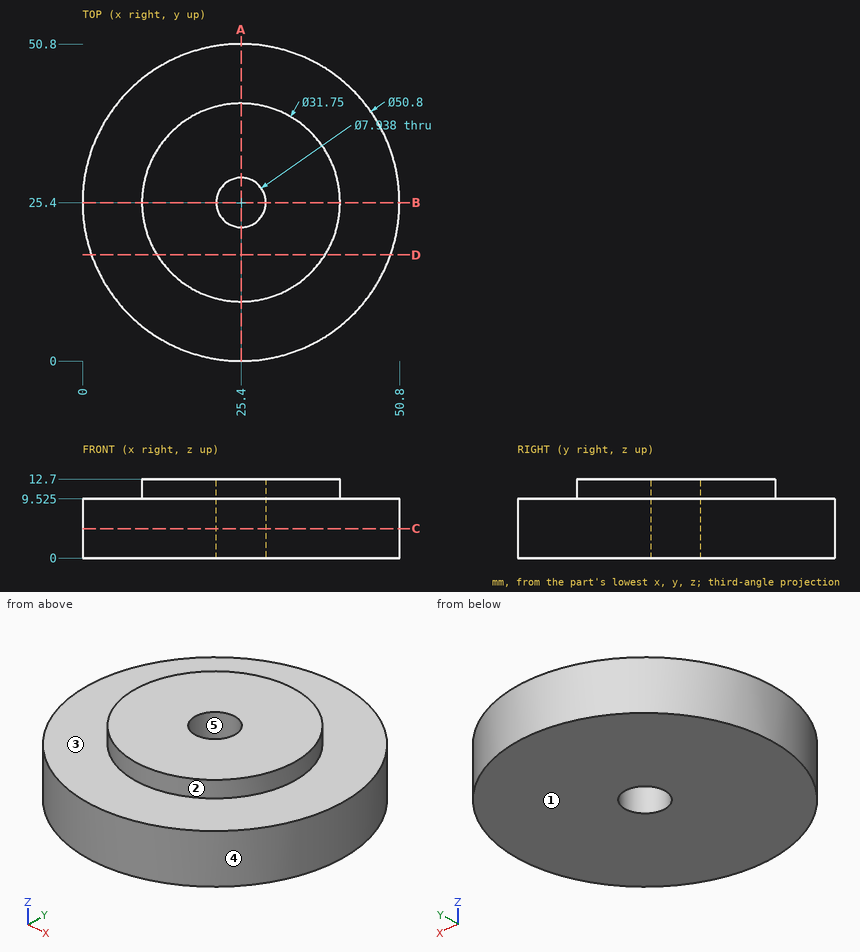
Print and shaded views of the part. All mm, measured from the part's lowest x, y and z. A direction names the side the tool comes from. Coordinates: 2 decimals unless noted, no trailing zeros. Order: outer loops, then holes, each group sorted by start corner. A loop starts at its lowest first (then second) coordinate and runs counter-clockwise, first axis right, second up. Notation, with made-up numbers: (-11.5, 38) - (33.5, 38) arc R27 cw to (33.5, 54) - close; hole circle Ø9 at (62, 49). An arc over 180 degrees is marked (long way). Return JSON: item names as keys, results as strings. Group by question number.
Item 1: Pin check, flat tips, straight feed: pin 1 (3 mm diameter, centred on x = 8.5, z = 7.5, fed in from -Y); pin 2 (1 mm diameter, centred on x = 26, z = 10.5, fed in from -Y) (1 decimal); pin 3 (5 mm diameter, centred on y = 39.5, z = 3.5, fed in from +X). Stop position of each tip, or through.
Item 2: Cut at C-C (z = 4.75). List the corners of the cut face in (x, y).
Item 3: Cut at D-D (y = 17). List the corners of the cut face in (x, z) (1 decimal).
Item 4: Which spindle directions (+Z, -Z, +X, -X, +Y, -Y) get a long thin tool onto all of the face, cutting with end or side? Do the marked faces 1 and 2. Say none if no direction does.
Item 5: Pull direction Y, two halves, no side cores. Call the marked faces 3, 4 and 5: pulls with the +Y half, pulls with the -Y half, needs draft (parallel to the pull), parting line crosses it, or undercut.
Item 6: Drill centre lines: probe 1 along Y at (x, z) = (25.4, 3.25); probe 2 along Z at (x, y) = (47, 31.5) (1 decimal); probe 3 along Y at (x, z) = (25.4, 10) (1 decimal). Where is each one in solid material? Low to high. Write a range as from..to.
Item 7: Cut at A-A (x = 25.4). List the corners of the cut face in (y, z) (1 decimal).
Check values:
{
 "1": {"pin 1": "stops at y = 5.2", "pin 2": "stops at y = 9.5", "pin 3": "stops at x = 48"},
 "2": {"outline": "circle Ø50.8 at (25.4, 25.4); hole circle Ø7.94 at (25.4, 25.4)"},
 "3": {"outline": "(1.4, 0) - (49.4, 0) - (49.4, 9.5) - (38.9, 9.5) - (38.9, 12.7) - (11.9, 12.7) - (11.9, 9.5) - (1.4, 9.5) - close"},
 "4": {"face 1": "-Z, +X, -X, +Y, -Y", "face 2": "+Z"},
 "5": {"face 3": "needs draft", "face 4": "parting line crosses it", "face 5": "undercut"},
 "6": {"probe 1": "y = 0..21.43, 29.37..50.8", "probe 2": "z = 0..9.5", "probe 3": "y = 9.5..21.4, 29.4..41.3"},
 "7": {"outline": "(0, 0) - (21.4, 0) - (21.4, 12.7) - (9.5, 12.7) - (9.5, 9.5) - (0, 9.5) - close; (29.4, 0) - (50.8, 0) - (50.8, 9.5) - (41.3, 9.5) - (41.3, 12.7) - (29.4, 12.7) - close"}
}
